Source: three-view drawing plus pictorial views. Frame: mm from the lowest corner of the part. A direction names the side the tool comes from. Give positions to 0.01 mm unless a question says otherwise; leave off trailing zeros. Loops run counter-clockwise (first coordinate to the right, second up) from the corner with the lowest first, then second, coordinate; pieces in that order, holes last. Notation, with made-up numbers: (-35.75, -40) -> (-30.75, -40) arc R22 ccw to (-30.75, -28) -> close; hole circle Ø7 at (74.5, -40). An arc over 180 degrees is marked (long way). Answer as a JSON object with one key per item and string values. Group by question number.
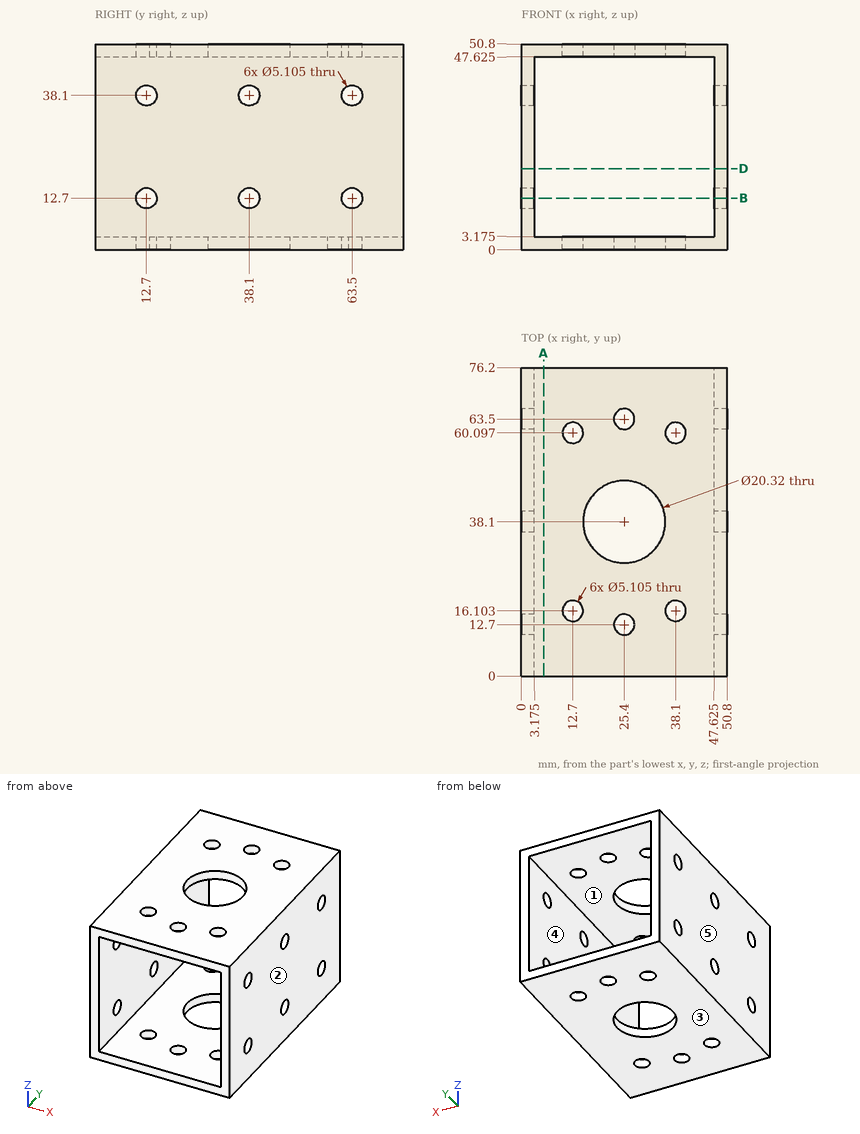
(1) Section query D-D on z = 20. Return the cut outline in (x, y) (1 decimal), plus the area to 3 significant figures.
(2) Material intervals for line 1 (Z direction, x = 2.05, y = 38.1); line 2 (Y direction, x = 48, z = 38); line 3 (Z direction, x = 27, y = 22.5) (1 decimal), sorted ascending. Write a range as from..to.
(3) Access query for the marked faces 1 and 2. Directions: +Z, -Z, +X, -X, +Y, -Y. A direction counts if a zero-diameter tool reaches every point of the face in a straight line with its end or side. Return the directions, or none.
(4) Mould query, pull axis Z, two halves, no side actions, for the marked faces 3, 4 and 5. Classes: pulls with the +Z half, pulls with the -Z half, needs draft (parallel to the pull), parting line crosses it, or undercut.
(5) Section query A-A on x = 5.5. Return the cut outline in (y, z) (1 decimal).
(6) First-contact query: pin 1 (4.5 mm diameter, centred on x = 38.1, y = 60.1, fed in from -Z). Flat tip, straight axial feed; report the tip coordinate or a pass-through.
(7) Section query B-B on z = 12.7. State how many separate pieces and enclosed holes the cut face has.
Result:
{
 "1": {"outline": "(0, 0) -> (3.2, 0) -> (3.2, 76.2) -> (0, 76.2) -> close; (47.6, 0) -> (50.8, 0) -> (50.8, 76.2) -> (47.6, 76.2) -> close", "area": "484 mm²"},
 "2": {"line 1": "0..10.15, 15.25..35.55, 40.65..50.8", "line 2": "0..10.15, 15.25..35.55, 40.65..60.95, 66.05..76.2", "line 3": "0..3.2, 47.6..50.8"},
 "3": {"face 1": "+Y, -Y", "face 2": "+Z, -Z, +X, +Y, -Y"},
 "4": {"face 3": "pulls with the -Z half", "face 4": "undercut", "face 5": "needs draft"},
 "5": {"outline": "(0, 0) -> (76.2, 0) -> (76.2, 3.2) -> (0, 3.2) -> close; (0, 47.6) -> (76.2, 47.6) -> (76.2, 50.8) -> (0, 50.8) -> close"},
 "6": {"pin 1": "through"},
 "7": {"separate pieces": "8", "enclosed holes": "0"}
}
